Source: CAD feature listing. Evaluate the final solid. Frame: model axes, mm. Face numbers are marked on the shaded views. Round coordinates to 2 decimals unless told otherwise and drop trailing zeros. Loops run counter-clockwise (first coordinate to the right, second up) from the corner with the lowest first, then second, coordinate; pieces in that order, holes last. Notation, with made-up numbers: (68.5, -19.75) -> (122.5, -19.75) arc R19 cw to (122.5, 2.25) -> close; hole circle Ø3 at (83.5, 3.25). An arc over 180 degrees is marked (long way). Put each result on its own line as item: value. Start each with the question number.
1. Cut plane C-C (x = -15). Return the cut outline in (y, z).
2. Cut plane A-A (y = 13). Return the cut outline in (x, z).
3. Cut plane B-B (z = 0). Return the cut outline in (x, y), then the cut area to 3 significant figures.
4. Contact query for flat-ended pins moving along their axis: pin 1 (0.6 mm diameter, centred on y = 1.5, z = 52.5, fed in from -X); pin 2 (1 mm diameter, centred on x = -2.5, y = 1, fed in from -Z); pin 3 (7.5 mm diameter, centred on y = 8, z = 38, fed in from +X). Output: stop coordinate, or through.
5. Draft query along Z for the marked faces 1 and 2. Return one class per face: pulls with the +Z half, pulls with the -Z half, needs draft (parallel to the pull), parting line crosses it, or undercut.
6. Material intervals for L1, parallel to X at y = 1.5, z = 0; L2, parallel to Z at x = 3, y = 15.25; L3, parallel to X at y = 7, z = 39.5, sorted ascending.
7. Cut plane D-D (z = 33). Return the cut outline in (x, y), then the cut area to 3 significant figures.
```python
from build123d import *

# Parameters (mm, degrees)
SKETCH1_R           = 57
BOSS_EXTRUDE1_DEPTH = 2
BOSS_EXTRUDE2_DEPTH = 1
SKETCH3_W           = 16.631913854
SKETCH3_H           = 33
SKETCH3_W_2         = 12.5
SKETCH3_H_2         = 23
BOSS_EXTRUDE3_DEPTH = 15
SKETCH4_W           = 10
SKETCH4_H           = 10.084358196
CUT_EXTRUDE1_DEPTH  = 20
SKETCH5_W           = 17.04328316
SKETCH5_H           = 4.71779089
CUT_EXTRUDE2_DEPTH  = 20
SKETCH6_R           = 2.5
CUT_EXTRUDE3_DEPTH  = 20


with BuildPart() as part:
    # Sketch1 → Boss-Extrude1 (new body)
    with BuildSketch(Plane(origin=(0, 0, 0), x_dir=(1, 0, 0), z_dir=(0, 1, 0))):
        with Locations(Location((0, 0, 0), (0, 0, 270))):
            Circle(SKETCH1_R)
    extrude(amount=BOSS_EXTRUDE1_DEPTH)

    # Sketch2 → Boss-Extrude2 (add)
    with BuildSketch(Plane(origin=(0, 2, 0), x_dir=(1, 0, 0), z_dir=(0, 1, 0))):
        with BuildLine():
            Line((-56.568542495, 7), (-50.986982029, 6.30931713))
            ThreePointArc((-50.986982029, 6.30931713), (-46.729900776, 21.34938389), (-38.147214926, 34.413221478))
            Line((-38.147214926, 34.413221478), (-42.323202173, 38.180447324))
            ThreePointArc((-42.323202173, 38.180447324), (-51.84543726, 23.686507453), (-56.568542495, 7))
        make_face()
        with BuildLine():
            Line((42.323202173, 38.180447324), (38.147214926, 34.413221478))
            ThreePointArc((38.147214926, 34.413221478), (46.729900776, 21.34938389), (50.986982029, 6.30931713))
            Line((50.986982029, 6.30931713), (56.568542495, 7))
            ThreePointArc((56.568542495, 7), (51.84543726, 23.686507453), (42.323202173, 38.180447324))
        make_face()
        with BuildLine():
            Line((56.568542495, -7), (50.986982029, -6.30931713))
            ThreePointArc((50.986982029, -6.30931713), (46.729900776, -21.34938389), (38.147214926, -34.413221478))
            Line((38.147214926, -34.413221478), (42.323202173, -38.180447324))
            ThreePointArc((42.323202173, -38.180447324), (51.84543726, -23.686507453), (56.568542495, -7))
        make_face()
        with BuildLine():
            Line((-42.323202173, -38.180447324), (-38.147214926, -34.413221478))
            ThreePointArc((-38.147214926, -34.413221478), (-46.729900776, -21.34938389), (-50.986982029, -6.30931713))
            Line((-50.986982029, -6.30931713), (-56.568542495, -7))
            ThreePointArc((-56.568542495, -7), (-51.84543726, -23.686507453), (-42.323202173, -38.180447324))
        make_face()
    extrude(amount=BOSS_EXTRUDE2_DEPTH)

    # Sketch3 → Boss-Extrude3 (add)
    with BuildSketch(Plane(origin=(0, 2, 0), x_dir=(1, 0, 0), z_dir=(0, 1, 0))):
        with Locations((0, 32.5)):
            Rectangle(SKETCH3_W, SKETCH3_H)
        with Locations((0, 33.5)):
            Rectangle(SKETCH3_W_2, SKETCH3_H_2, mode=Mode.SUBTRACT)
    boss_extrude3 = extrude(amount=BOSS_EXTRUDE3_DEPTH)

    # Sketch4 → Cut-Extrude1 (cut)
    with BuildSketch(Plane(origin=(0, 0, -49), x_dir=(-1, 0, 0), z_dir=(0, 0, -1))):
        with Locations((0, 9.671309809)):
            Rectangle(SKETCH4_W, SKETCH4_H)
    cut_extrude1 = extrude(amount=-CUT_EXTRUDE1_DEPTH, mode=Mode.SUBTRACT)

    # Sketch5 → Cut-Extrude2 (cut)
    with BuildSketch(Plane(origin=(0, 2, 0), x_dir=(1, 0, 0), z_dir=(0, 1, 0))):
        with Locations((0, 52.127337333)):
            Rectangle(SKETCH5_W, SKETCH5_H)
    cut_extrude2 = extrude(amount=-CUT_EXTRUDE2_DEPTH, mode=Mode.SUBTRACT)

    # Mirror1: Boss-Extrude3, Cut-Extrude1, Cut-Extrude2 across plane
    add(boss_extrude3.mirror(Plane.XY))
    add(cut_extrude1.mirror(Plane.XY), mode=Mode.SUBTRACT)
    add(cut_extrude2.mirror(Plane.XY), mode=Mode.SUBTRACT)

    # Sketch6 → Cut-Extrude3 (cut)
    with BuildSketch(Plane(origin=(0, 2, 0), x_dir=(1, 0, 0), z_dir=(0, 1, 0))):
        with Locations(Location((-10, 0, 0), (0, 0, 270))):
            Circle(SKETCH6_R)
        with Locations(Location((0, 10, 0), (0, 0, 270))):
            Circle(SKETCH6_R)
        with Locations(Location((10, 0, 0), (0, 0, 270))):
            Circle(SKETCH6_R)
        with Locations(Location((0, -10, 0), (0, 0, 270))):
            Circle(SKETCH6_R)
        with BuildLine():
            Line((-21.172323644, 39.708093778), (-11.762402025, 22.060052099))
            ThreePointArc((-11.762402025, 22.060052099), (-25, 0), (-11.762402025, -22.060052099))
            Line((-11.762402025, -22.060052099), (-21.172323644, -39.708093778))
            ThreePointArc((-21.172323644, -39.708093778), (-45, 0), (-21.172323644, 39.708093778))
        make_face()
        with BuildLine():
            Line((21.172323644, 39.708093778), (11.762402025, 22.060052099))
            ThreePointArc((11.762402025, 22.060052099), (25, 0), (11.762402025, -22.060052099))
            Line((11.762402025, -22.060052099), (21.172323644, -39.708093778))
            ThreePointArc((21.172323644, -39.708093778), (45, 0), (21.172323644, 39.708093778))
        make_face()
    extrude(amount=-CUT_EXTRUDE3_DEPTH, mode=Mode.SUBTRACT)


solid = part.part
```
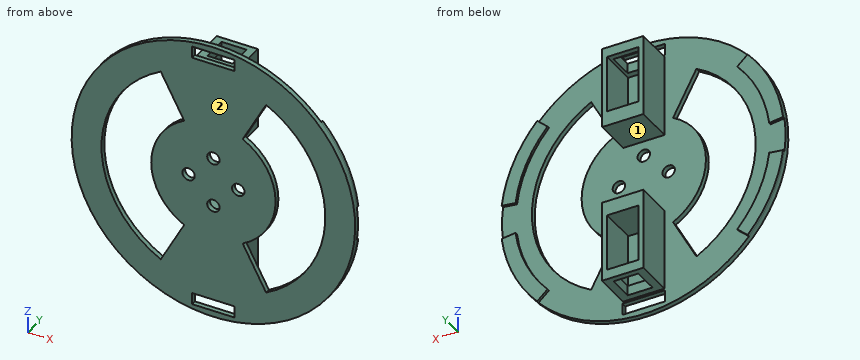
Solution:
1. outline: (0, -54.99) -> (2, -54.99) -> (2, -28.13) -> (0, -28.13) -> close; (0, -20) -> (2, -20) -> (2, 20) -> (0, 20) -> close; (0, 28.13) -> (2, 28.13) -> (2, 54.99) -> (0, 54.99) -> close
2. outline: (-8.32, -49) -> (-5, -49) -> (-5, -45) -> (-6.25, -45) -> (-6.25, -22) -> (6.25, -22) -> (6.25, -45) -> (5, -45) -> (5, -49) -> (8.32, -49) -> (8.32, -16) -> (-8.32, -16) -> close; (-8.32, 16) -> (8.32, 16) -> (8.32, 49) -> (5, 49) -> (5, 45) -> (6.25, 45) -> (6.25, 22) -> (-6.25, 22) -> (-6.25, 45) -> (-5, 45) -> (-5, 49) -> (-8.32, 49) -> close
3. outline: (-57, 0) -> (-45, 0) -> (-45, 2) -> (-57, 2) -> close; (-25, 0) -> (-12.5, 0) -> (-12.5, 2) -> (-25, 2) -> close; (-7.5, 0) -> (7.5, 0) -> (7.5, 2) -> (-7.5, 2) -> close; (12.5, 0) -> (25, 0) -> (25, 2) -> (12.5, 2) -> close; (45, 0) -> (57, 0) -> (57, 2) -> (45, 2) -> close
3. area: 128 mm^2
4. pin 1: stops at x = -22.89
4. pin 2: stops at z = -56.96
4. pin 3: stops at x = 8.32
5. face 1: undercut
5. face 2: needs draft
6. L1: x = -57 to -45, -25 to -12.5, -7.5 to 7.5, 12.5 to 25, 45 to 57
6. L2: z = -49 to -45, -22 to -16, 16 to 22, 45 to 49
6. L3: x = -8.32 to -6.25, 6.25 to 8.32
7. outline: (-46.48, 0) -> (-30.59, 0) -> (-30.59, 2) -> (-39.38, 2) -> (-39.38, 3) -> (-46.48, 3) -> close; (-17.6, 0) -> (17.6, 0) -> (17.6, 2) -> (8.32, 2) -> (8.32, 17) -> (6.25, 17) -> (6.25, 2) -> (-6.25, 2) -> (-6.25, 17) -> (-8.32, 17) -> (-8.32, 2) -> (-17.6, 2) -> close; (30.59, 0) -> (46.48, 0) -> (46.48, 3) -> (39.38, 3) -> (39.38, 2) -> (30.59, 2) -> close
7. area: 210 mm^2
